Source: three-view drawing plus pictorial views. Frame: mm from the lowest corner of the part. Give positions to 0.01 mm unless a question says otherwise; leave off trailing zeros. Loops run counter-clockwise (first coordinate to the right, second up) from the corner with the lowest first, then second, coordinate; pieces in that order, holes last. Notation, with made-up numbers: (45.5, 56) - (94.5, 56) arc R7 cw to (94.5, 61) - close; hole circle Ø8 at (65.5, 29.25). An arc over 180 degrees is marked (long way). Answer in a Markdown table with one row per item.
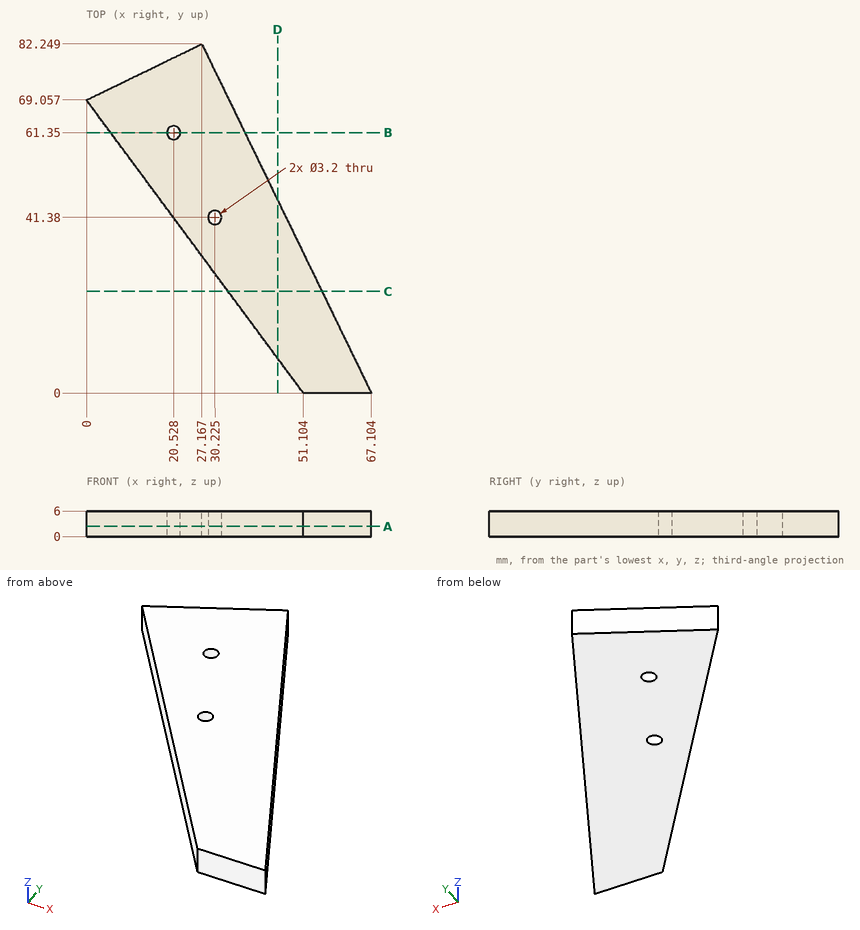
Q1. Cut plane D-D (x = 45). Output: boundary loops of the cut face in (y, z).
Check values:
| item | result |
|---|---|
| outline | (8.25, 0) - (45.52, 0) - (45.52, 6) - (8.25, 6) - close |
Q2. Cut plane C-C (y = 24). Output: boundary loops of the cut face in (x, z).
Check values:
| item | result |
|---|---|
| outline | (33.34, 0) - (55.45, 0) - (55.45, 6) - (33.34, 6) - close |
Q3. Material intervals for line 1 along X through (y, z) = (28, 5) (1 decimal); line 2 along Y through (x, z) = (35, 3.6) (1 decimal); line 3 along X through (y, z) = (77, 5.65) (1 decimal), sorted ascending.
Check values:
| item | result |
|---|---|
| line 1 | 30.4 to 53.5 |
| line 2 | 21.8 to 66.1 |
| line 3 | 16.4 to 29.7 |
Q4. First-contact query: pin 1 (10 mm diameter, centred on x = 12.5, y = 45, fed in from +Z); pin 2 (3 mm diameter, centred on y = 13, z = 2.5, fed in from +X); pin 3 (1 mm diameter, centred on x = 11, z = 4, fed in from +Y). Flat tips, straight axial feed; report the tip coordinate or a pass-through.
Check values:
| item | result |
|---|---|
| pin 1 | z = 6 |
| pin 2 | x = 61.52 |
| pin 3 | y = 74.64 |
Q5. Cut plane B-B (y = 61.35). Output: boundary loops of the cut face in (x, z) (1 decimal).
Check values:
| item | result |
|---|---|
| outline | (5.7, 0) - (18.9, 0) - (18.9, 6) - (5.7, 6) - close; (22.1, 0) - (37.3, 0) - (37.3, 6) - (22.1, 6) - close |
Q6. Cut plane A-A (z = 2.4). Give the number of separate pieces and of enclosed holes in the cut face, and give its area (3 significant figures).
Check values:
| item | result |
|---|---|
| separate pieces | 1 |
| enclosed holes | 2 |
| area | 1,920 mm² |
